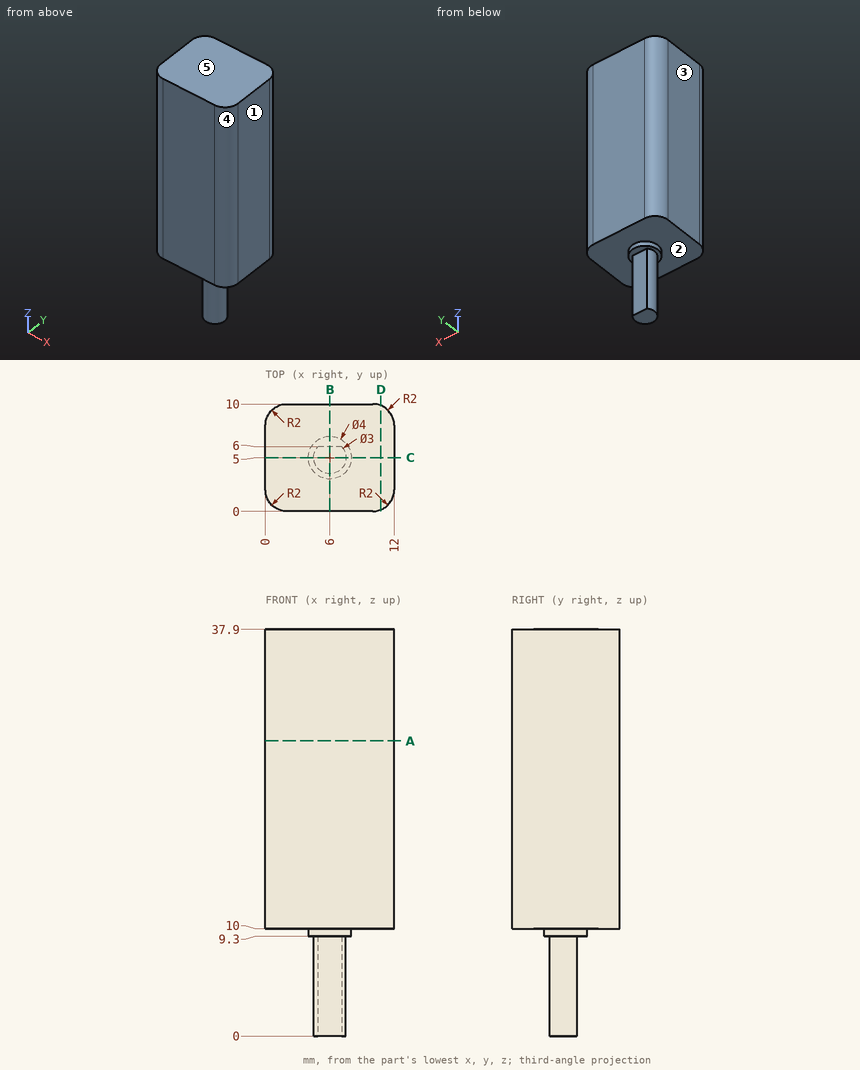
Geometry: see drawing. Coordinates: mm, zero at the bounding-box minimum. A direction names the side the tool comes from. Give positions to 0.01 mm unless a question says otherwise; leave off trailing zeros. Order: outer loops, then holes, each group sorted by start corner. A loop starts at its lowest first (then second) coordinate and runs counter-clockwise, first axis right, second up. Notation, with made-up numbers: M 22.5,76 L 65.5,76 A14 cw 65.5,96 Z; hole C 33.5,-30.5 d3. An arc over 180 degrees is marked long. Answer as a JSON object with one key per item and string values.
1. Cut plane A-A, the plane z = 27.5. Output: boundary loops of the cut face in (x, y).
Result sheet:
{"outline": "M 0,2 A2 ccw 2,0 L 10,0 A2 ccw 12,2 L 12,8 A2 ccw 10,10 L 2,10 A2 ccw 0,8 Z"}
2. First-contact query: P1, Ø1.1, axis at x = 5.5, z = 6, coming from the +Y side. Flat tip, straight axial feed; report the tip coordinate or a pass-through.
Result sheet:
{"P1": "y = 6"}
3. Cut plane D-D, the plane x = 10.75. Output: boundary loops of the cut face in (y, z).
Result sheet:
{"outline": "M 0.15,10 L 9.85,10 L 9.85,37.9 L 0.15,37.9 Z"}
4. Cut plane B-B, the plane x = 6. Output: boundary loops of the cut face in (y, z), and give its area (3 significant figures).
Result sheet:
{"outline": "M 0,10 L 3,10 L 3,9.3 L 3.5,9.3 L 3.5,0 L 6,0 L 6,9.3 L 7,9.3 L 7,10 L 10,10 L 10,37.9 L 0,37.9 Z", "area": "305 mm²"}
5. Reachability of the marked faces 1 and 2 from +Z, -Z, +X, -X, +Y, -Y: full face, straight path, thin tool, end or side. Return the list, or none.
Result sheet:
{"face 1": "+Z, -Z, +X, +Y, -Y", "face 2": "-Z"}
6. Pull-direction query (X, two-part tool) for the marked faces 3, 4 and 5; classes: +X half, -X half, draft (parallel to the pull), parting line (faces both ways), or undercut.
Result sheet:
{"face 3": "-X half", "face 4": "+X half", "face 5": "draft"}
7. Cut plane C-C, the plane y = 5. Output: boundary loops of the cut face in (x, z).
Result sheet:
{"outline": "M 0,10 L 4,10 L 4,9.3 L 4.5,9.3 L 4.5,0 L 7.5,0 L 7.5,9.3 L 8,9.3 L 8,10 L 12,10 L 12,37.9 L 0,37.9 Z"}
8. Ray query, line 1 (Z direction, x = 4.75, y = 2); line 2 (X direction, y = 1.5, z = 15); line 3 (Y direction, x = 1, z = 23.5). Return the intervals inside material, ascending. Write a range as [from, to].
Result sheet:
{"line 1": "[10, 37.9]", "line 2": "[0.06, 11.94]", "line 3": "[0.27, 9.73]"}
